Can you work these out from the model? Positions are in its coordinate system, mm. Face numbers are marked on the shaded views. Coordinates: 2 decimals unless noted, no trailing zeros. Order: outer loops, then holes, each group sorted by start corner. A loop starts at its lowest first (then second) coordinate and runs counter-clockwise, first axis right, second up. Notation, with made-up numbers: (71, 31.25) -> (76, 31.25) arc R25 ccw to (76, 67.25) -> close; hole circle Ø2 at (11, 55.25). An arc over 180 degrees is marked (long way). Use a Markdown table: item, result. Add a question column.
1. Suppose I cut it at D-D, the plane x = 4.25. List the corners of the cut face in (y, z) for me.
2. Suppose I cut it at C-C, the plane x = 0. List the corners of the cut face in (y, z) for me.
3. Suppose I cut it at A-A, the plane z = 0. List the corners of the cut face in (x, y) for me.
4. Suppose I cut it at B-B, the plane y = 7.5. List the corners of the cut face in (x, z) for me.
5. If I drill on line 1 along X through (y, z) = (7.5, -4.75); line 2 along Y through (x, z) = (6, 0), over which ranges is the centre line in solid material (lowest first)? Write a range as from..to.
6. We'd pull the mould along Y, two halves only. Please class the marked faces 1, 2, 3 and 4: pulls with the +Y half, pulls with the -Y half, needs draft (parallel to the pull), parting line crosses it, or undercut.
```python
from build123d import *

# Parameters (mm, degrees)
SKETCH_1_W      = 15
SKETCH_1_H      = 15
EXTRUDE_1_DEPTH = 15
M5X0_8_1_D      = 4.2
M5X0_8_2_D      = 4.2
M5X0_8_3_D      = 4.2
CHAMFER_1_SIZE  = 0.1


with BuildPart() as part:
    # 草图1 → 凸台-拉伸1 (new body)
    with BuildSketch(Plane(origin=(0, 0, 0), x_dir=(1, 0, 0), z_dir=(0, 1, 0))):
        Rectangle(SKETCH_1_W, SKETCH_1_H)
    extrude(amount=EXTRUDE_1_DEPTH)

    # M5x0.8 螺纹孔1 (through all)
    with Locations(Plane(origin=(0, 15, 0), x_dir=(1, 0, 0), z_dir=(0, 1, 0))):
        with Locations((0, 0)):
            Hole(M5X0_8_1_D / 2)

    # M5x0.8 螺纹孔2 (through all)
    with Locations(Plane(origin=(0, 0, -7.5), x_dir=(-1, 0, 0), z_dir=(0, 0, -1))):
        with Locations((0, 7.5)):
            Hole(M5X0_8_2_D / 2)

    # M5x0.8 螺纹孔3 (through all)
    with Locations(Plane.ZY.offset(7.5)):
        with Locations((0, 7.5)):
            Hole(M5X0_8_3_D / 2)

    # 倒角1
    chamfer_1_edges = [part.edges().sort_by_distance(p)[0] for p in [
        (-7.5, 15, 0),
        (7.5, 15, 0),
        (0, 0, 7.5),
        (-7.5, 0, 0),
        (0, 0, -7.5),
        (7.5, 0, 0),
        (7.5, 7.5, 7.5),
        (-7.5, 7.5, 7.5),
        (-7.5, 7.5, -7.5),
        (7.5, 7.5, -7.5),
        (0, 15, -7.5),
    ]]
    chamfer(chamfer_1_edges, length=CHAMFER_1_SIZE)


solid = part.part
```
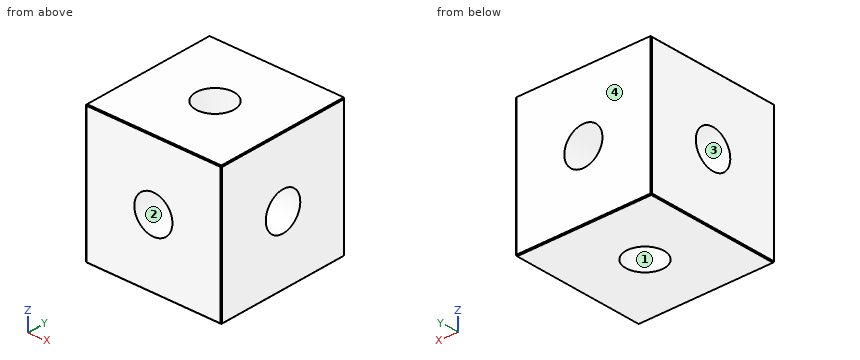
Worked out:
| question | item | result |
|---|---|---|
| 1 | outline | (0, -7.4) -> (0.1, -7.5) -> (14.9, -7.5) -> (15, -7.4) -> (15, 7.5) -> (0.1, 7.5) -> (0, 7.4) -> close; hole circle Ø4.2 at (7.5, 0) |
| 2 | outline | (0, -7.4) -> (0.1, -7.5) -> (5.4, -7.5) -> (5.4, -2.1) -> (0, -2.1) -> close; (0, 2.1) -> (5.4, 2.1) -> (5.4, 7.5) -> (0.1, 7.5) -> (0, 7.4) -> close; (9.6, -7.5) -> (14.9, -7.5) -> (15, -7.4) -> (15, -2.1) -> (9.6, -2.1) -> close; (9.6, 2.1) -> (15, 2.1) -> (15, 7.5) -> (9.6, 7.5) -> close |
| 3 | outline | (-7.5, 0.1) -> (-7.4, 0) -> (-2.1, 0) -> (-2.1, 5.4) -> (-7.5, 5.4) -> close; (-7.5, 9.6) -> (-2.1, 9.6) -> (-2.1, 15) -> (-7.4, 15) -> (-7.5, 14.9) -> close; (2.1, 0) -> (7.4, 0) -> (7.5, 0.1) -> (7.5, 5.4) -> (2.1, 5.4) -> close; (2.1, 9.6) -> (7.5, 9.6) -> (7.5, 14.9) -> (7.4, 15) -> (2.1, 15) -> close |
| 4 | outline | (-7.5, -7.4) -> (-7.4, -7.5) -> (-2.1, -7.5) -> (-2.1, -2.1) -> (-7.5, -2.1) -> close; (-7.5, 2.1) -> (-2.1, 2.1) -> (-2.1, 7.5) -> (-7.4, 7.5) -> (-7.5, 7.4) -> close; (2.1, -7.5) -> (7.4, -7.5) -> (7.5, -7.4) -> (7.5, -2.1) -> (2.1, -2.1) -> close; (2.1, 2.1) -> (7.5, 2.1) -> (7.5, 7.4) -> (7.4, 7.5) -> (2.1, 7.5) -> close |
| 5 | line 1 | x = -7.5..-2.1, 2.1..7.5 |
| 5 | line 2 | y = 0..5.4, 9.6..15 |
| 6 | face 1 | undercut |
| 6 | face 2 | needs draft |
| 6 | face 3 | undercut |
| 6 | face 4 | pulls with the +Y half |
